```python
from build123d import *

# Parameters (mm, degrees)
SKETCH3_W           = 56
SKETCH3_H           = 21
BOSS_EXTRUDE1_DEPTH = 130
SKETCH4_W           = 52
SKETCH4_H           = 106
SKETCH4_H_2         = 20
CUT_EXTRUDE3_DEPTH  = 22
SKETCH6_R           = 1.5
SKETCH6_R_2         = 1.25
CUT_EXTRUDE4_DEPTH  = 57
FILLET1_R           = 10
SKETCH7_W           = 80
SKETCH7_H           = 10
CUT_EXTRUDE5_DEPTH  = 57
SKETCH8_W           = 36
SKETCH8_H           = 10
CUT_EXTRUDE6_DEPTH  = 2
CUT_EXTRUDE7_DEPTH  = 57


with BuildPart() as part:
    # Sketch3 → Boss-Extrude1 (new body)
    with BuildSketch(Plane.XY):
        Rectangle(SKETCH3_W, SKETCH3_H)
    extrude(amount=BOSS_EXTRUDE1_DEPTH)

    # Sketch4 → Cut-Extrude3 (cut, through all)
    with BuildSketch(Plane.XZ.offset(10.5)):
        with Locations((0, 53)):
            Rectangle(SKETCH4_W, SKETCH4_H)
        with Locations((0, 117.5)):
            Rectangle(SKETCH4_W, SKETCH4_H_2)
    extrude(amount=-CUT_EXTRUDE3_DEPTH, mode=Mode.SUBTRACT)

    # Sketch6 → Cut-Extrude4 (cut, through all)
    with BuildSketch(Plane(origin=(28, 0, 0), x_dir=(0, 0, -1), z_dir=(1, 0, 0))):
        with Locations((-12, 0)):
            Circle(SKETCH6_R)
        with Locations((-4.5, 0)):
            Circle(SKETCH6_R_2)
        with Locations((-19.5, 0)):
            Circle(SKETCH6_R_2)
        with Locations((-12, 7.5)):
            Circle(SKETCH6_R_2)
        with Locations((-12, -7.5)):
            Circle(SKETCH6_R_2)
    extrude(amount=-CUT_EXTRUDE4_DEPTH, mode=Mode.SUBTRACT)

    # Fillet1
    fillet1_edges = [part.edges().sort_by_distance(p)[0] for p in [
        (27, -10.5, 0),
        (-27, 10.5, 0),
        (-27, -10.5, 0),
        (27, 10.5, 0),
    ]]
    fillet(fillet1_edges, radius=FILLET1_R)

    # Sketch7 → Cut-Extrude5 (cut, through all)
    with BuildSketch(Plane(origin=(28, 0, 0), x_dir=(0, 0, -1), z_dir=(1, 0, 0))):
        with Locations((-65, -0.5)):
            Rectangle(SKETCH7_W, SKETCH7_H)
    extrude(amount=-CUT_EXTRUDE5_DEPTH, mode=Mode.SUBTRACT)

    # Sketch8 → Cut-Extrude6 (cut)
    with BuildSketch(Plane(origin=(0, 0, 106), x_dir=(-1, 0, 0), z_dir=(0, 0, -1))):
        Rectangle(SKETCH8_W, SKETCH8_H)
    extrude(amount=-CUT_EXTRUDE6_DEPTH, mode=Mode.SUBTRACT)

    # Sketch9 → Cut-Extrude7 (cut, through all)
    with BuildSketch(Plane(origin=(28, 0, 0), x_dir=(0, 0, -1), z_dir=(1, 0, 0))):
        Polygon((8.328518313, 0), (-140.648225394, 0), (-140.648225394, 18.171038809), (9.8749897, 18.171038809), (9.8749897, 0), align=None)
    extrude(amount=-CUT_EXTRUDE7_DEPTH, mode=Mode.SUBTRACT)


solid = part.part
```
The listing builds one solid part. Answer for the finished solid, in the listing's coordinates (mm). A direction names the side the tool comes from. Give positions to 0.01 mm unless a question says otherwise; leave off trailing zeros. Order: outer loops, then holes, each group sorted by start corner. A loop starts at its lowest first (then second) coordinate and runs counter-clockwise, first axis right, second up. Notation, with made-up numbers: M 28,-31.75 L 76,-31.75 A23 ccw 76,5.25 Z; hole C 44.5,-0.5 d3. An arc over 180 degrees is marked long. Put each result on its own line as item: value. Start each with the question number.
Item 1: The part is cut by section D-D, the plane z = 12. Determine the outline of the cut face in (x, y), and give its area (3 significant figures).
Item 2: For a pull along Z with two mould halves and no side action, classify faces 4 (the face through (27.01, -8.26, 12.99)), 5 (the face through (0, 0, 128)), 6 (the face through (27.01, -7.65, 3.01)) as +Z half, -Z half, draft (parallel to the pull), parting line (faces both ways), or undercut.
Item 3: Flat-ended cylindrical pins translate along their axes: P1, Ø0.8, axis at x = -4.5, z = 107, coming from the +Y side; P2, Ø1, axis at x = 26.5, y = -2.5, coming from the -Z side; P3, Ø1.5, axis at y = -7.5, z = 12, coming from the +X side; P4, Ø3, axis at x = -4, y = -5, coming from the -Z side. Find the tip coordinate at first contact, or state that the pin passes through.
Item 4: Which of the six approach directions +Z, -Z, +X, -X, +Y, -Y give full straight-line access (tool end or side, diameter ignored) to faces 1 (the face through (0, -5, 127.5)), 2 (the face through (28, -6, 64)), 3 (the face through (26, -8, 40))?
Item 5: The part is cut by section A-A, the plane x = 21. Determine the outline of the cut face in (y, z), and give its area (3 significant figures).
Item 6: The part is cut by section B-B, the plane z = 95. Determine the outline of the cut face in (x, y).
Item 7: The part is cut by section C-C, the plane y = -7.5. Determine the outline of the cut face in (x, z).
Item 8: Find the intervals of material crossed by line 1 along X through (y, z) = (-3.5, 109); line 2 along Z through (x, y) = (6, -9.25); line 3 along Y through (x, z) = (27.15, 12), in increasing order.
Answer key:
1. outline: M -28,-10.5 L -26,-10.5 L -26,-8.75 L -28,-8.75 Z; M -28,-6.25 L -26,-6.25 L -26,-1.5 L -28,-1.5 Z; M 26,-10.5 L 28,-10.5 L 28,-8.75 L 26,-8.75 Z; M 26,-6.25 L 28,-6.25 L 28,-1.5 L 26,-1.5 Z
1. area: 26.0 mm²
2. face 4: undercut
2. face 5: draft
2. face 6: -Z half
3. P1: stops at y = -5
3. P2: stops at z = 0.11
3. P3: passes through
3. P4: stops at z = 106
4. face 1: +Y, -Y
4. face 2: +Z, -Z, +X, +Y, -Y
4. face 3: -Z, +Y, -Y
5. outline: M -10.5,106 L 0,106 L 0,107.5 L -10.5,107.5 Z; M -10.5,127.5 L 0,127.5 L 0,130 L -10.5,130 Z
5. area: 42.0 mm²
6. outline: M -28,-10.5 L -26,-10.5 L -26,-5.5 L -28,-5.5 Z; M 26,-10.5 L 28,-10.5 L 28,-5.5 L 26,-5.5 Z
7. outline: M -28,2.86 L -26,2.86 L -26,10.75 L -28,10.75 Z; M -28,13.25 L -26,13.25 L -26,106 L 26,106 L 26,13.25 L 28,13.25 L 28,130 L -28,130 Z; M 26,2.86 L 28,2.86 L 28,10.75 L 26,10.75 Z; hole M -26,107.5 L 26,107.5 L 26,127.5 L -26,127.5 Z
8. line 1: x = -28 to -26, 26 to 28
8. line 2: z = 106 to 107.5, 127.5 to 130
8. line 3: y = -10.5 to -8.75, -6.25 to -1.5
